Could you check a few things on this model? Use its own coordinates, in mm. Face numbers are marked on the shaded views. A direction names the side the tool comes from. Round coordinates to 2 decimals unless told otherwise and drop trailing zeros. Loops run counter-clockwise (first coordinate to the right, second up) from the corner with the lowest first, then second, coordinate; pieces in that order, holes last. Notation, with made-up numbers: (67, 14) -> (93, 14) arc R34 ccw to (93, 52) -> close; hole circle Ø1 at (-39, 80.25). An arc over 180 degrees is marked (long way). One line per item, written item: value.
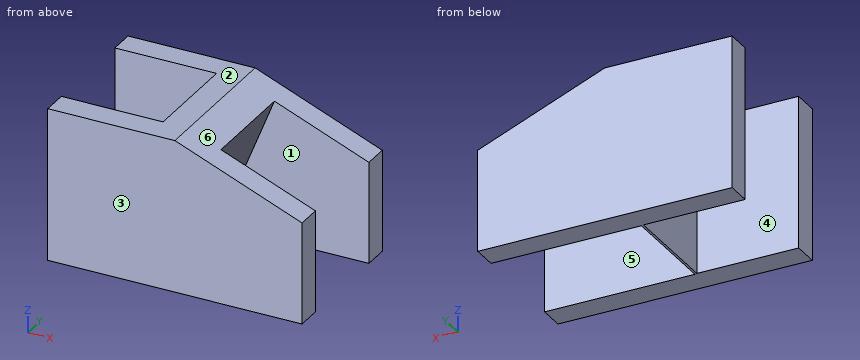
from build123d import *

# Parameters (mm, degrees)
F1_DEPTH = 76.2
F2_W     = 50.8
F2_H     = 50.8
F3_DEPTH = 94.234
F4_W     = 50.8
F4_H     = 134.9397847399
F5_DEPTH = 41.656
F6_W     = 50.8
F6_H     = 50.8
F7_DEPTH = 88.138


with BuildPart() as f1:
    # F0 (on Front) → F1 (new body)
    with BuildSketch(Plane.XZ):
        Polygon((-79.544827342, 62.9425281554), (-79.544827342, -13.2574718446), (47.455172658, -13.2574718446), (47.455172658, 37.5425281554), (-16.044827342, 62.9425281554), align=None)
    extrude(amount=F1_DEPTH)

    # F2 (on face) → F3 (cut)
    with BuildSketch(Plane(origin=(19.4912404202, 0, 48.7281010505), x_dir=(0.9284766909, 0, -0.3713906764), z_dir=(0.3713906764, 0, 0.9284766909))):
        with Locations((4.7180767512, -38.1)):
            Rectangle(F2_W, F2_H)
    extrude(amount=-F3_DEPTH, mode=Mode.SUBTRACT)

    # F4 (on face) → F5 (cut)
    with BuildSketch(Plane(origin=(27.9639322377, 0, -11.1855728951), x_dir=(0, -1, 0), z_dir=(-0.9284766909, 0, 0.3713906764))):
        with Locations((38.1, 65.2383889087)):
            Rectangle(F4_W, F4_H)
    extrude(amount=-F5_DEPTH, mode=Mode.SUBTRACT)

    # F6 (on face) → F7 (cut)
    with BuildSketch(Plane.XY.offset(62.9425281554)):
        with Locations((-54.144827342, -37.8712617517)):
            Rectangle(F6_W, F6_H)
    extrude(amount=-F7_DEPTH, mode=Mode.SUBTRACT)


solid = f1.part
(1) If we section it at C-C, the plane z = 23.5: Please give me the cut outline in (x, y).
Recorded:
outline: (-79.54, -76.2) -> (47.46, -76.2) -> (47.46, -63.5) -> (-12.88, -63.5) -> (-12.88, -12.7) -> (47.46, -12.7) -> (47.46, 0) -> (-79.54, 0) -> (-79.54, -12.47) -> (-28.74, -12.47) -> (-28.74, -63.27) -> (-79.54, -63.27) -> close
(2) If we section it at B-B, the plane y = -45: Please give me the cut outline in (x, z).
Recorded:
outline: (-28.74, -13.26) -> (-27.58, -13.26) -> (0.29, 56.41) -> (-16.04, 62.94) -> (-28.74, 62.94) -> close
(3) For the marked faces 4, 5 and 6, which set-ups out of +Z, -Z, +X, -X, +Y, -Y let a thin tool reach every point of the face, with its end or its side?
Recorded:
face 4: +Z, -Z, -X
face 5: -Z, +X
face 6: +Z, +X, +Y, -Y
(4) I'm going to push flat-ended pins straight in: pin 1 Ø5 at (x, y) = (-2, -23) entering from -Z; pin 2 Ø1 at (y, z) = (-40, 19.5) entering from +X; pin 3 Ø12 at (y, z) = (-27.5, 51) entering from -X. Where does each tip first touch, or does it pass through?
Recorded:
pin 1: z = 44.44
pin 2: x = -14.28
pin 3: x = -28.74
(5) Thinking about a two-plate mould opening in Y: for the marked faces 1, 2 and 3, which applies, released by +Y, released by -Y, zero draft, split by the parting line, or undercut?
Recorded:
face 1: undercut
face 2: zero draft
face 3: released by -Y
(6) If we section it at D-D, the plane x = -8: Please give me the cut outline in (y, z).
Recorded:
outline: (-76.2, -13.26) -> (-63.5, -13.26) -> (-63.5, 35.69) -> (-12.7, 35.69) -> (-12.7, -13.26) -> (0, -13.26) -> (0, 59.72) -> (-76.2, 59.72) -> close
(7) If I drill on L1, parallel to Y at x = -8.5, z = 21.5; L2, parallel to Y at x = -66, z = -6.5; L3, parallel to X at y = -43, z = 22.5, over which ranges is the centre line in solid material (lowest first)?
Recorded:
L1: -76.2 to -63.5, -12.7 to 0
L2: -76.2 to -63.27, -12.47 to 0
L3: -28.74 to -13.28
(8) If we section it at A-A, the plane x = -40.5: Please give me the cut outline in (y, z), then the cut area to 3 significant figures.
Recorded:
outline: (-76.2, -13.26) -> (-63.27, -13.26) -> (-63.27, 62.94) -> (-76.2, 62.94) -> close; (-12.47, -13.26) -> (0, -13.26) -> (0, 62.94) -> (-12.47, 62.94) -> close
area: 1,940 mm²
